```python
from build123d import *

# Parameters (mm, degrees)
BOSS_EXTRUDE1_DEPTH = 3
SKETCH2_W           = 3
SKETCH2_H           = 1
CUT_EXTRUDE1_DEPTH  = 10


with BuildPart() as part:
    # Sketch1 → Boss-Extrude1 (new body)
    with BuildSketch(Plane.XY):
        with BuildLine():
            Line((1.5, 6.891), (-1.5, 6.891))
            Line((-1.5, 6.891), (-3.462838736, 9.995543944))
            Line((-3.462838736, 9.995543944), (-5.270057432, 8.366602698))
            Line((-5.270057432, 8.366602698), (-2.022319198, 4.380080358))
            Line((-2.022319198, 4.380080358), (-2.462490424, 3.788964217))
            Line((-2.462490424, 3.788964217), (-4.816528245, 5.541884903))
            Line((-4.816528245, 5.541884903), (-8.240611079, 3.54862106))
            ThreePointArc((-8.240611079, 3.54862106), (-12.719726234, -3.813407871), (-5.642674559, -8.730447848))
            Line((-5.642674559, -8.730447848), (-1.5, -6.614))
            Line((-1.5, -6.614), (-1.5, 0))
            Line((-1.5, 0), (1.5, 0))
            Line((1.5, 0), (1.5, -6.614))
            Line((1.5, -6.614), (5.642674559, -8.730447848))
            ThreePointArc((5.642674559, -8.730447848), (12.719726234, -3.813407871), (8.240611079, 3.54862106))
            Line((8.240611079, 3.54862106), (4.816528245, 5.541884903))
            Line((4.816528245, 5.541884903), (2.462490424, 3.788964217))
            Line((2.462490424, 3.788964217), (2.022319198, 4.380080358))
            Line((2.022319198, 4.380080358), (5.270057432, 8.366602698))
            Line((5.270057432, 8.366602698), (3.462838736, 9.995543944))
            Line((3.462838736, 9.995543944), (1.5, 6.891))
        make_face()
    extrude(amount=-BOSS_EXTRUDE1_DEPTH)

    # Sketch2 → Cut-Extrude1 (cut)
    with BuildSketch(Plane.XY):
        with Locations((0, 0.5)):
            Rectangle(SKETCH2_W, SKETCH2_H)
    extrude(amount=-CUT_EXTRUDE1_DEPTH, mode=Mode.SUBTRACT)


solid = part.part
```
Read the model definition and answer for the solid it produces. Units are mm, in the model's axes. A direction names the side the tool comes from. Give positions to 0.01 mm unless a question says otherwise; leave off trailing zeros. Order: outer loops, then holes, each group sorted by start corner. A loop starts at its lowest first (then second) coordinate and runs counter-clockwise, first axis right, second up. Notation, with made-up numbers: (15, -28.75) -> (20, -28.75) arc R17 ccw to (20, -20.75) -> close; hole circle Ø6 at (6.5, 36). An arc over 180 degrees is marked (long way). One line per item, written item: value. Start each with the question number.
(1) The part is cut by section C-C (z = -1.2). Determine the outline of the cut face in (x, y).
(2) The part is cut by section B-B (x = 4.5). Determine the outline of the cut face in (y, z), and give its area (3 significant figures).
(3) For a pull along Y with two mould halves and no side action, classify faces 1 (the flat face through (1.5, -3, -1)), 2 (the flat face through (-3.67, 6.4, -1.48)), 3 (the flat face through (4.38, 9.17, -1.48)), 4 (the cylindrical face through (12.7, -3.9, -1.5)) as released by +Y, released by -Y, zero draft, split by the parting line, or undercut.
(4) A tool of negligible diameter and unlimited length cuts with its end or side. For faces 5 (the flat face through (0, 6.891, -1)), 6 (the flat face through (-3, -1, -3)), 7 (the flat face through (-1.5, -3, -1)), 8 (the flat face through (-3.62, 4.65, -1.48)), 9 (the flat face through (-4.354, 9.192, -1.479)), from which of +Z, -Z, +X, -X, +Y, -Y can it reach the whole face along a straight path? Write none if from no direction.
(5) Straight lines are drawn through the part: L1, parallel to Y at x = -3.25, z = -2.55; L2, parallel to X at y = -1.5, z = -2.4; L3, parallel to Y at x = -2.75, z = -1.65. For each, find the intervals that lie inside material, in ascending order.
(6) The part is cut by section D-D (x = 0.5). Determine the outline of the cut face in (y, z).
(7) A flat-ended cylindrical pin translates along its axis: P1, Ø1.5, axis at y = -2, z = -2, coming from the +X side. Find the tip coordinate at first contact, or state that the pin passes through.
(8) The part is cut by section A-A (y = -2). Determine the outline of the cut face in (x, z) (3 decimals), and give its area (3 significant figures).
Taken from the geometry:
1. outline: (-8.24, 3.55) arc R6.29 ccw to (-5.64, -8.73) -> (-1.5, -6.61) -> (-1.5, 1) -> (1.5, 1) -> (1.5, -6.61) -> (5.64, -8.73) arc R6.29 ccw to (8.24, 3.55) -> (4.82, 5.54) -> (2.46, 3.79) -> (2.02, 4.38) -> (5.27, 8.37) -> (3.46, 10) -> (1.5, 6.89) -> (-1.5, 6.89) -> (-3.46, 10) -> (-5.27, 8.37) -> (-2.02, 4.38) -> (-2.46, 3.79) -> (-4.82, 5.54) -> close
2. outline: (-8.15, -3) -> (5.31, -3) -> (5.31, 0) -> (-8.15, 0) -> close; (7.42, -3) -> (9.06, -3) -> (9.06, 0) -> (7.42, 0) -> close
2. area: 45.3 mm^2
3. face 1: zero draft
3. face 2: undercut
3. face 3: released by +Y
3. face 4: split by the parting line
4. face 5: +Z, -Z, +Y
4. face 6: -Z, +X, -X, +Y, -Y
4. face 7: +Z, -Z, -Y
4. face 8: +Z, -Z
4. face 9: +Z, -Z, -X, +Y
5. L1: -7.51 to 4.38, 5.89 to 9.66
5. L2: -12.77 to -1.5, 1.5 to 12.77
5. L3: -7.25 to 4, 5.27 to 8.87
6. outline: (1, -3) -> (6.89, -3) -> (6.89, 0) -> (1, 0) -> close
7. P1: x = 12.86
8. outline: (-12.835, -3) -> (-1.5, -3) -> (-1.5, 0) -> (-12.835, 0) -> close; (1.5, -3) -> (12.835, -3) -> (12.835, 0) -> (1.5, 0) -> close
8. area: 68.0 mm^2
